```python
from build123d import *

# Parameters (mm, degrees)
SKETCH004_W     = 61.15
SKETCH004_H     = 54.8
PAD001_DEPTH    = 20
POCKET003_DEPTH = 61.151
SKETCH006_R     = 3.34
SKETCH006_W     = 16.51
SKETCH006_H     = 11
POCKET004_DEPTH = 5
SKETCH007_R     = 3.34
SKETCH007_W     = 15.2570581741
SKETCH007_H     = 10.1100032783
POCKET005_DEPTH = 17
SKETCH008_W     = 23
SKETCH008_H     = 23
SKETCH008_R     = 10.5
PAD002_DEPTH    = 40
POCKET006_DEPTH = 61.151
PAD004_DEPTH    = 2


with BuildPart() as part:
    # Sketch004 → Pad001 (new body)
    with BuildSketch(Plane.XY):
        with Locations((4.8749828339, -3.3899418259)):
            Rectangle(SKETCH004_W, SKETCH004_H)
    extrude(amount=PAD001_DEPTH)

    # Sketch005 (on Face2 of Pad001) → Pocket003 (cut, through all)
    with BuildSketch(Plane.YZ.offset(35.4499828339)):
        Polygon((-30.7899418259, 20), (-0.7899418259, 20), (-30.7899418259, 6), align=None)
    extrude(amount=-POCKET003_DEPTH, mode=Mode.SUBTRACT)

    # Sketch006 (on Face3 of Pocket003) → Pocket004 (cut)
    with BuildSketch(Plane.YZ.offset(35.4499828339)):
        with Locations((-8.7709418259, -0.3499967217)):
            Circle(SKETCH006_R)
        with Locations((-21.8049418259, 0.1500032783)):
            Circle(SKETCH006_R)
        with Locations((6.7920581741, 4.6100032783)):
            Rectangle(SKETCH006_W, SKETCH006_H)
    extrude(amount=-POCKET004_DEPTH, mode=Mode.SUBTRACT)

    # Sketch007 (on Face2 of Pocket004) → Pocket005 (cut)
    with BuildSketch(Plane(origin=(-25.7000171661, 0, 0), x_dir=(0, -1, 0), z_dir=(-1, 0, 0))):
        with Locations((21.8049418259, -0.8499967217)):
            Circle(SKETCH007_R)
        with Locations((-7.6285290871, 5.0550016391)):
            Rectangle(SKETCH007_W, SKETCH007_H)
    extrude(amount=-POCKET005_DEPTH, mode=Mode.SUBTRACT)

    # Sketch008 (on Face5 of Pocket005) → Pad002 (join)
    with BuildSketch(Plane.XY.offset(20)):
        with Locations((5.2999828339, 12.2100581741)):
            Rectangle(SKETCH008_W, SKETCH008_H)
        with Locations((5.2999828339, 12.2100581741)):
            Circle(SKETCH008_R, mode=Mode.SUBTRACT)
    extrude(amount=PAD002_DEPTH)

    # Sketch010 (on Face3 of Pocket005) → Pocket006 (cut, through all)
    with BuildSketch(Plane.YZ.offset(35.4499828339)):
        Polygon((-28.7899418259, 0), (-28.7899418259, 4.6), (-0.7899418259, 18), (22.0100581741, 18), (22.0100581741, 0), align=None)
    extrude(amount=-POCKET006_DEPTH, mode=Mode.SUBTRACT)

    # Sketch011 (on Face2 of Pocket006) → Pad004 (join)
    with BuildSketch(Plane(origin=(-25.7000171661, 0, 0), x_dir=(0, -1, 0), z_dir=(-1, 0, 0))):
        with BuildLine():
            Line((-22.0100581741, 0), (-22.0100581741, 18))
            Line((-22.0100581741, 18), (0.7899418259, 18))
            Line((0.7899418259, 18), (28.7899418259, 4.6))
            Line((28.7899418259, 4.6), (28.7899418259, 0))
            Line((24.8049418259, 0), (28.7899418259, 0))
            ThreePointArc((24.8049418259, 0), (21.8049418259, 2.2680947501), (18.8049418259, 0))
            Line((1.4629418259, 0), (18.8049418259, 0))
            Line((1.4629418259, 10.1100032783), (1.4629418259, 0))
            Line((-15.2570581741, 10.1100032783), (1.4629418259, 10.1100032783))
            Line((-15.2570581741, 0), (-15.2570581741, 10.1100032783))
            Line((-22.0100581741, 0), (-15.2570581741, 0))
        make_face()
    extrude(amount=-PAD004_DEPTH)


with BuildPart() as part_1:
    # Body001 placement: moved
    add(part.part.moved(Location((0, 0, 10))))


solid = part_1.part
```
Work out the finished part from the listing and answer in its coordinate system (mm). A direction names the side the tool comes from. Coordinates: 2 decimals unless noted, no trailing zeros. Write each loop counter-clockwise with the first axis right and the second up, starting at its lowest first coordinate (ties: lowest second). Pieces come first, ordered by that corner, then holes. Notation, with made-up numbers: (-38, -30) - (-16, -30) arc R17 ccw to (-16, -19) - close; hole circle Ø11 at (-7, -19.5). An arc over 180 degrees is marked (long way). Answer as a JSON object with one key per item and string values.
Q1. Find section D-D (z = 25). Write down the section's boundary in (x, y), plus the area to 3 significant figures.
Results list:
{"outline": "(-25.7, -11.5) - (35.45, -11.5) - (35.45, -7.06) - (-23.7, -7.06) - (-23.7, 22.01) - (35.45, 22.01) - (35.45, 24.01) - (-25.7, 24.01) - close", "area": "452 mm^2"}
Q2. Given pin 1 Ø14.5 at (y, z) = (3, 18) entering from +X; pin 2 Ø6 at (x, y) = (-13, 10.5) entering from -Z; pin 3 Ø10 at (x, z) = (-11, 50.5) entering from -Y, each flat-ended and moving along its own axis, determine where each tip first touches the part or whether it passes through.
Results list:
{"pin 1": "stops at x = -23.7", "pin 2": "stops at z = 28", "pin 3": "stops at y = 0.71"}
Q3. For a pull along Y with two mould halves and no side action, classify faces 4 (the flat face through (4, 24.01, 20)), 5 (the flat face through (2, -30, 10)), 6 (the flat face through (6.3, -15, 21.2)), 7 (the flat face through (5.3, -15.58, 23.1)) as pulls with the +Y half, pulls with the -Y half, needs draft (parallel to the pull), parting line crosses it, or undercut.
Results list:
{"face 4": "pulls with the +Y half", "face 5": "needs draft", "face 6": "undercut", "face 7": "pulls with the -Y half"}
Q4. Consider L1, parallel to Y at x = 4.5, z = 14; L2, parallel to Z at x = 14.5, y = 14; L3, parallel to Y at x = -11.5, z = 15. Determine where each line is inside the solid, lowest interval first. Write a range as from..to.
Results list:
{"L1": "y = -30.79..-28.79, 22.01..24.01", "L2": "z = 28..30", "L3": "y = -30.79..-27.95, 22.01..24.01"}
Q5. Find section C-C (y = 6.5). Write down the section's boundary in (x, z), plus the area to 3 significant figures.
Results list:
{"outline": "(-25.7, 20.11) - (-23.7, 20.11) - (-23.7, 28) - (35.45, 28) - (35.45, 30) - (16.8, 30) - (16.8, 70) - (14.11, 70) - (14.11, 30) - (-3.51, 30) - (-3.51, 70) - (-6.2, 70) - (-6.2, 30) - (-25.7, 30) - close", "area": "353 mm^2"}
Q6. Find section A-A (x = -16). Write down the section's boundary in (y, z).
Results list:
{"outline": "(-30.79, 10) - (-28.79, 10) - (-28.79, 14.6) - (-0.79, 28) - (22.01, 28) - (22.01, 10) - (24.01, 10) - (24.01, 30) - (-0.79, 30) - (-30.79, 16) - close"}
Q7. Find section B-B (z = 31.5). Write down the section's boundary in (x, y).
Results list:
{"outline": "(-6.2, 0.71) - (16.8, 0.71) - (16.8, 23.71) - (-6.2, 23.71) - close; hole circle Ø21 at (5.3, 12.21)"}
Q8. Which of the six approach directions +Z, -Z, +X, -X, +Y, -Y give full straight-line access (tool end or side, diameter ignored) to faces 1 (the flat face through (5, 23.71, 50)), 2 (the flat face through (-25, 7, 20.11)), 3 (the flat face through (-23.7, -4, 19))?
Results list:
{"face 1": "+Z, +X, -X, +Y", "face 2": "-Z, +X, -X", "face 3": "-Z, +X"}
